from build123d import *

# Parameters (mm, degrees)
F0_R     = 19.939
F1_DEPTH = 6.35
F2_R     = 15.875
F3_DEPTH = 12.7
F4_R     = 9.525
F5_DEPTH = 25.4
F7_DEPTH = 25.4


with BuildPart() as f1:
    # F0 (on Top) → F1 (new body)
    with BuildSketch(Plane.XY):
        Circle(F0_R)
    extrude(amount=F1_DEPTH)

    # F2 (on face) → F3 (join)
    with BuildSketch(Plane.XY.offset(6.35)):
        Circle(F2_R)
    extrude(amount=F3_DEPTH)

    # F4 (on face) → F5 (cut)
    with BuildSketch(Plane.XY.offset(19.05)):
        Circle(F4_R)
    extrude(amount=-F5_DEPTH, mode=Mode.SUBTRACT)

    # F6 (on face) → F7 (cut)
    with BuildSketch(Plane.XY.offset(6.35)):
        with BuildLine():
            Line((-2.5334230713, 19.777398427), (-1.5679899251, 17.5945175959))
            ThreePointArc((-1.5679899251, 17.5945175959), (0, 16.5735), (1.5679899251, 17.5945175959))
            Line((1.5679899251, 17.5945175959), (2.5334230713, 19.777398427))
            ThreePointArc((2.5334230713, 19.777398427), (0, 19.939), (-2.5334230713, 19.777398427))
        make_face()
        with BuildLine():
            ThreePointArc((9.1449076101, 17.7181936383), (6.8195396378, 18.7365311659), (4.3836296792, 19.4511570822))
            Line((4.3836296792, 19.4511570822), (4.5442508678, 17.0697224901))
            ThreePointArc((4.5442508678, 17.0697224901), (5.6684708454, 15.5739956506), (7.491107992, 15.9971542122))
            Line((7.491107992, 15.9971542122), (9.1449076101, 17.7181936383))
        make_face()
        with BuildLine():
            ThreePointArc((14.6533813266, 13.521913204), (12.8165421495, 15.2741601513), (10.7719519949, 16.7788191247))
            Line((10.7719519949, 16.7788191247), (10.1083879401, 14.4860669297))
            ThreePointArc((10.1083879401, 14.4860669297), (10.6532404491, 12.696037578), (12.5106878781, 12.4702979377))
            Line((12.5106878781, 12.4702979377), (14.6533813266, 13.521913204))
        make_face()
        with BuildLine():
            ThreePointArc((18.3944409942, 7.6946904752), (17.2676805261, 9.9695), (15.8610179229, 12.0827079518))
            Line((15.8610179229, 12.0827079518), (14.4533042428, 10.155177906))
            ThreePointArc((14.4533042428, 10.155177906), (14.3530720296, 8.28675), (16.0212941679, 7.4393396899))
            Line((16.0212941679, 7.4393396899), (18.3944409942, 7.6946904752))
        make_face()
        with BuildLine():
            ThreePointArc((19.9168596049, 0.9393745136), (19.6360817873, 3.4623710145), (19.0370110058, 5.9292438781))
            Line((19.0370110058, 5.9292438781), (17.0549387459, 4.5994245523))
            ThreePointArc((17.0549387459, 4.5994245523), (16.3217112945, 2.8779580726), (17.5994959321, 1.5110872826))
            Line((17.5994959321, 1.5110872826), (19.9168596049, 0.9393745136))
        make_face()
        with BuildLine():
            ThreePointArc((19.0370110058, -5.9292438781), (19.6360817873, -3.4623710145), (19.9168596049, -0.9393745136))
            Line((19.9168596049, -0.9393745136), (17.5994959321, -1.5110872826))
            ThreePointArc((17.5994959321, -1.5110872826), (16.3217112945, -2.8779580726), (17.0549387459, -4.5994245523))
            Line((17.0549387459, -4.5994245523), (19.0370110058, -5.9292438781))
        make_face()
        with BuildLine():
            ThreePointArc((15.8610179229, -12.0827079518), (17.2676805261, -9.9695), (18.3944409942, -7.6946904752))
            Line((18.3944409942, -7.6946904752), (16.0212941679, -7.4393396899))
            ThreePointArc((16.0212941679, -7.4393396899), (14.3530720296, -8.28675), (14.4533042428, -10.155177906))
            Line((14.4533042428, -10.155177906), (15.8610179229, -12.0827079518))
        make_face()
        with BuildLine():
            ThreePointArc((10.7719519949, -16.7788191247), (12.8165421495, -15.2741601513), (14.6533813266, -13.521913204))
            Line((14.6533813266, -13.521913204), (12.5106878781, -12.4702979377))
            ThreePointArc((12.5106878781, -12.4702979377), (10.6532404491, -12.696037578), (10.1083879401, -14.4860669297))
            Line((10.1083879401, -14.4860669297), (10.7719519949, -16.7788191247))
        make_face()
        with BuildLine():
            ThreePointArc((4.3836296792, -19.4511570822), (6.8195396378, -18.7365311659), (9.1449076101, -17.7181936383))
            Line((9.1449076101, -17.7181936383), (7.491107992, -15.9971542122))
            ThreePointArc((7.491107992, -15.9971542122), (5.6684708454, -15.5739956506), (4.5442508678, -17.0697224901))
            Line((4.5442508678, -17.0697224901), (4.3836296792, -19.4511570822))
        make_face()
        with BuildLine():
            Line((-1.5679899251, -17.5945175959), (-2.5334230713, -19.777398427))
            ThreePointArc((-2.5334230713, -19.777398427), (0, -19.939), (2.5334230713, -19.777398427))
            Line((2.5334230713, -19.777398427), (1.5679899251, -17.5945175959))
            ThreePointArc((1.5679899251, -17.5945175959), (0, -16.5735), (-1.5679899251, -17.5945175959))
        make_face()
        with BuildLine():
            Line((-7.491107992, -15.9971542122), (-9.1449076101, -17.7181936383))
            ThreePointArc((-9.1449076101, -17.7181936383), (-6.8195396378, -18.7365311659), (-4.3836296792, -19.4511570822))
            Line((-4.3836296792, -19.4511570822), (-4.5442508678, -17.0697224901))
            ThreePointArc((-4.5442508678, -17.0697224901), (-5.6684708454, -15.5739956506), (-7.491107992, -15.9971542122))
        make_face()
        with BuildLine():
            Line((-12.5106878781, -12.4702979377), (-14.6533813266, -13.521913204))
            ThreePointArc((-14.6533813266, -13.521913204), (-12.8165421495, -15.2741601513), (-10.7719519949, -16.7788191247))
            Line((-10.7719519949, -16.7788191247), (-10.1083879401, -14.4860669297))
            ThreePointArc((-10.1083879401, -14.4860669297), (-10.6532404491, -12.696037578), (-12.5106878781, -12.4702979377))
        make_face()
        with BuildLine():
            Line((-16.0212941679, -7.4393396899), (-18.3944409942, -7.6946904752))
            ThreePointArc((-18.3944409942, -7.6946904752), (-17.2676805261, -9.9695), (-15.8610179229, -12.0827079518))
            Line((-15.8610179229, -12.0827079518), (-14.4533042428, -10.155177906))
            ThreePointArc((-14.4533042428, -10.155177906), (-14.3530720296, -8.28675), (-16.0212941679, -7.4393396899))
        make_face()
        with BuildLine():
            Line((-17.5994959321, -1.5110872826), (-19.9168596049, -0.9393745136))
            ThreePointArc((-19.9168596049, -0.9393745136), (-19.6360817873, -3.4623710145), (-19.0370110058, -5.9292438781))
            Line((-19.0370110058, -5.9292438781), (-17.0549387459, -4.5994245523))
            ThreePointArc((-17.0549387459, -4.5994245523), (-16.3217112945, -2.8779580726), (-17.5994959321, -1.5110872826))
        make_face()
        with BuildLine():
            Line((-17.0549387459, 4.5994245523), (-19.0370110058, 5.9292438781))
            ThreePointArc((-19.0370110058, 5.9292438781), (-19.6360817873, 3.4623710145), (-19.9168596049, 0.9393745136))
            Line((-19.9168596049, 0.9393745136), (-17.5994959321, 1.5110872826))
            ThreePointArc((-17.5994959321, 1.5110872826), (-16.3217112945, 2.8779580726), (-17.0549387459, 4.5994245523))
        make_face()
        with BuildLine():
            Line((-14.4533042428, 10.155177906), (-15.8610179229, 12.0827079518))
            ThreePointArc((-15.8610179229, 12.0827079518), (-17.2676805261, 9.9695), (-18.3944409942, 7.6946904752))
            Line((-18.3944409942, 7.6946904752), (-16.0212941679, 7.4393396899))
            ThreePointArc((-16.0212941679, 7.4393396899), (-14.3530720296, 8.28675), (-14.4533042428, 10.155177906))
        make_face()
        with BuildLine():
            Line((-10.1083879401, 14.4860669297), (-10.7719519949, 16.7788191247))
            ThreePointArc((-10.7719519949, 16.7788191247), (-12.8165421495, 15.2741601513), (-14.6533813266, 13.521913204))
            Line((-14.6533813266, 13.521913204), (-12.5106878781, 12.4702979377))
            ThreePointArc((-12.5106878781, 12.4702979377), (-10.6532404491, 12.696037578), (-10.1083879401, 14.4860669297))
        make_face()
        with BuildLine():
            Line((-4.5442508678, 17.0697224901), (-4.3836296792, 19.4511570822))
            ThreePointArc((-4.3836296792, 19.4511570822), (-6.8195396378, 18.7365311659), (-9.1449076101, 17.7181936383))
            Line((-9.1449076101, 17.7181936383), (-7.491107992, 15.9971542122))
            ThreePointArc((-7.491107992, 15.9971542122), (-5.6684708454, 15.5739956506), (-4.5442508678, 17.0697224901))
        make_face()
    extrude(amount=-F7_DEPTH, mode=Mode.SUBTRACT)


solid = f1.part
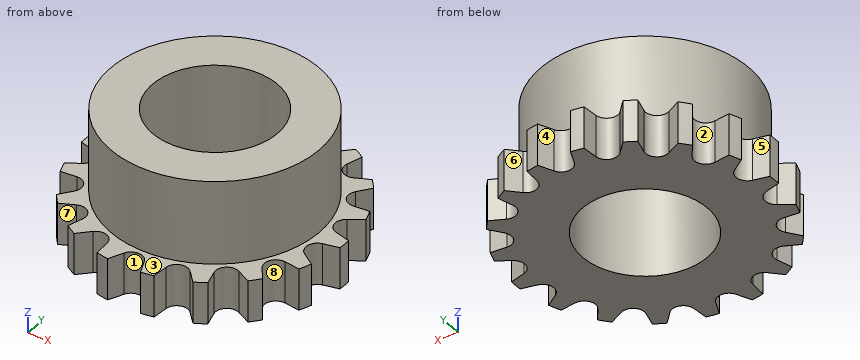
Design review of the part built by this model. Coordinates are the model's own, in mm. Face numbers are marked on the shaded views. A direction names the side the tool comes from. Round coordinates to 2 decimals unless told otherwise and drop trailing zeros. Write each loop counter-clockwise with the first axis right and the second up, starting at its lowest first coordinate (ties: lowest second). Pieces come first, ordered by that corner, then holes. Notation, with made-up numbers: M 13,69 L 21,69 A23 cw 21,79 Z; hole C -33.75,-8.75 d9. An arc over 180 degrees is marked long. One line per item, written item: value. Start each with the question number.
1. To check wall thickness, follow probe 1 along Y at (x, z) = (0, 4.5) (1 decimal); probe 2 along Y at (x, z) = (0, 9.25) (3 decimals); probe 3 along Z at (x, y) = (15, -13). State the ranges of each line that lie inside material, in increasing order. Write a range as from..to.
2. Take a section at C-C on z = 8.75. State the section outline as (x, y) points (3 decimals).
3. Clearance check with flat-ended pins moving along their axes: P1, Ø3, axis at y = 0.5, z = 15.5, coming from the +X side (3 decimals); P2, Ø1.5, axis at x = 1, z = 15, coming from the +Y side; P3, Ø3, axis at x = -15.5, z = 14.5, coming from the +Y side. State where each tip first meets the part, or that it passes through.
4. For the marked faces 5, 6, 7 and 8, list the 3-axis set-ups (+Z, -Z, +X, -X, +Y, -Y) from which the entire face can be reached by the end or side of a thin tool; tool diameter is ignored.
5. Draft analysis for pull direction Y (two halves, no side actions). For the marked faces 1, 2, 3 and 4, state which applies: pulls with the +Y half, pulls with the -Y half, needs draft (parallel to the pull), parting line crosses it, or undercut.
6. Take a section at B-B on y = 3.5. State the section outline as (x, z) points, then the cut area to 3 significant figures.
Computed:
1. probe 1: y = -16.6..-9.5, 9.5..16.6
1. probe 2: y = -15.875..-9.525, 9.525..15.875
1. probe 3: z = 0..6.35
2. outline: C 0,0 d31.75; hole C 0,0 d19.05
3. P1: stops at x = 15.875
3. P2: stops at y = 15.87
3. P3: stops at y = 7.48
4. face 5: +Z, -Z, -X
4. face 6: +Z, -Z, +Y
4. face 7: +Z, -Z, -Y
4. face 8: +Z, -Z
5. face 1: pulls with the -Y half
5. face 2: undercut
5. face 3: needs draft
5. face 4: pulls with the +Y half
6. outline: M -16.33,0 L -8.86,0 L -8.86,19.05 L -15.48,19.05 L -15.48,6.35 L -16.33,6.35 Z; M 8.86,0 L 16.33,0 L 16.33,6.35 L 15.48,6.35 L 15.48,19.05 L 8.86,19.05 Z
6. area: 263 mm²
